Geometry check sheet. Reference: drawing and pictorial views, mm from the part's lowest x, y, z. A direction names the side the tool comes from. Give positions to 0.01 mm unless a question says otherwise; leave off trailing zeros. Order: outer loops, then holes, each group sorted by start corner. A loop starts at its lowest first (then second) coordinate and runs counter-clockwise, first axis right, second up.
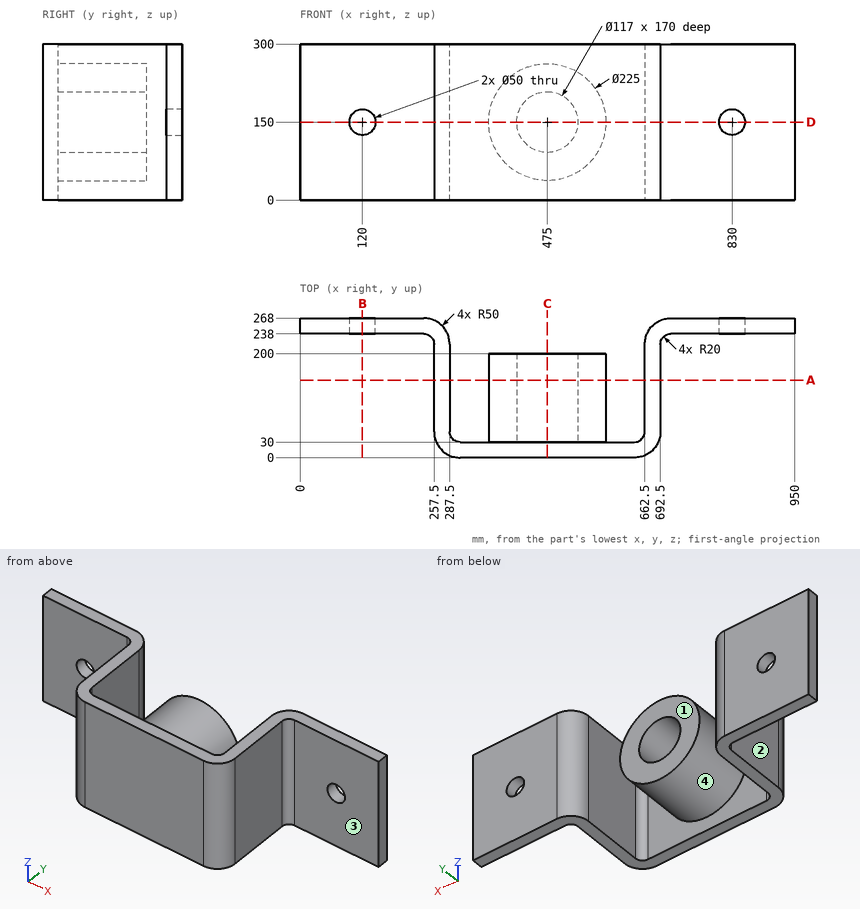
(1) Cross-section at C-C on x = 475. Enter the section's corners in (y, z), then the cut area to 3 significant figures.
Response values:
outline: (0, 0) - (30, 0) - (30, 37.5) - (200, 37.5) - (200, 91.5) - (30, 91.5) - (30, 208.5) - (200, 208.5) - (200, 262.5) - (30, 262.5) - (30, 300) - (0, 300) - close
area: 27,400 mm2
(2) Cross-section at B-B on x = 120. Enter the section's corners in (y, z), then the cut area to 3 significant figures.
Response values:
outline: (238, 0) - (268, 0) - (268, 125) - (238, 125) - close; (238, 175) - (268, 175) - (268, 300) - (238, 300) - close
area: 7,500 mm2
(3) Cross-section at D-D on z = 150. Count the separate pieces of the cut face and the enclosed holes in it, then the cut area to 3 significant figures.
Response values:
separate pieces: 3
enclosed holes: 0
area: 56,300 mm2
(4) Set-up check for the marked faces 1, 2, 3 and 4: record each of +Z, -Z, +X, -X, +Y, -Y from which the full face is reachable in a straight line by a thin tool's end or side.
Response values:
face 1: +Z, -Z, +Y
face 2: +Z, -Z, -X, -Y
face 3: +Z, -Z, +X, -Y
face 4: +Y
(5) Material ranges on L1, parallel to X at y = 140, z = 246; L2, parallel to X at y = 95.5, z = 150; L3, parallel to X at y = 159.5, z = 112, recorded low to high.
Response values:
L1: x = 257.5 to 287.5, 416.35 to 533.65, 662.5 to 692.5
L2: x = 257.5 to 287.5, 362.5 to 416.5, 533.5 to 587.5, 662.5 to 692.5
L3: x = 257.5 to 287.5, 369.11 to 430.52, 519.48 to 580.89, 662.5 to 692.5
(6) Cross-section at A-A on y = 149. Enter the section's corners in (x, z), then the cut area to 3 significant figures.
Response values:
outline: (257.5, 0) - (287.5, 0) - (287.5, 300) - (257.5, 300) - close; circle Ø225 at (475, 150); (662.5, 0) - (692.5, 0) - (692.5, 300) - (662.5, 300) - close; hole circle Ø117 at (475, 150)
area: 47,000 mm2
(7) Gauge pin test, flat ends, axial feed: pin 1 Ø2 at (y, z) = (200, 110) entering from -X; pin 2 Ø8 at (y, z) = (86.5, 130) entering from +X; pin 3 Ø1 at (x, y) = (482.5, 158.5) entering from -Z. Record the tip position at first contact, or that the pin passes through.
Response values:
pin 1: stops at x = 257.5
pin 2: stops at x = 692.5
pin 3: stops at z = 37.72
